For this review, take the finished solid that the model builds, in its own axes (mm). A direction names the side the tool comes from. Give positions to 0.01 mm unless a question says otherwise; leave off trailing zeros. Loops run counter-clockwise (first coordinate to the right, second up) from the corner with the lowest first, then second, coordinate; pieces in that order, holes last. Notation, with made-up numbers: (30.25, 19) - (50.25, 19) arc R20 cw to (50.25, 56) - close; hole circle Ø8 at (3.5, -23.75). An arc over 180 degrees is marked (long way). Answer in a Markdown table with one row per item.
```python
from build123d import *

# Parameters (mm, degrees)
BOSS_EXTRUDE2_DEPTH = 3
EXTRUDE_1_DEPTH     = 5
EXTRUDE_2_DEPTH     = 3


with BuildPart() as part:
    # Sketch3 → Boss-Extrude2 (new body)
    with BuildSketch(Plane.XY):
        with BuildLine():
            Line((-151, 81), (151, 81))
            ThreePointArc((151, 81), (158.071067812, 78.071067812), (161, 71))
            Line((161, 71), (161, -71))
            ThreePointArc((161, -71), (158.071067812, -78.071067812), (151, -81))
            Line((151, -81), (-151, -81))
            ThreePointArc((-151, -81), (-158.071067812, -78.071067812), (-161, -71))
            Line((-161, -71), (-161, 71))
            ThreePointArc((-161, 71), (-158.071067812, 78.071067812), (-151, 81))
        make_face()
    extrude(amount=-BOSS_EXTRUDE2_DEPTH)

    # Эскиз1 → Бобышка-Вытянуть1 (add)
    with BuildSketch(Plane(origin=(0, 0, -3), x_dir=(-1, 0, 0), z_dir=(0, 0, -1))):
        with BuildLine():
            Line((-151, -79), (151, -79))
            ThreePointArc((151, -79), (156.656854249, -76.656854249), (159, -71))
            Line((159, -71), (159, 71))
            ThreePointArc((159, 71), (156.656854249, 76.656854249), (151, 79))
            Line((151, 79), (-151, 79))
            ThreePointArc((-151, 79), (-156.656854249, 76.656854249), (-159, 71))
            Line((-159, 71), (-159, -71))
            ThreePointArc((-159, -71), (-156.656854249, -76.656854249), (-151, -79))
        make_face()
    extrude(amount=EXTRUDE_1_DEPTH)

    # Эскиз2 → Бобышка-Вытянуть2 (add)
    with BuildSketch(Plane.XY):
        with BuildLine():
            Line((-164.5, 71), (-151, 71))
            Line((-151, 71), (-151, 84.5))
            ThreePointArc((-151, 84.5), (-160.545941546, 80.545941546), (-164.5, 71))
        make_face()
        with BuildLine():
            Line((164.5, -71), (151, -71))
            Line((151, -71), (151, -84.5))
            ThreePointArc((151, -84.5), (160.545941546, -80.545941546), (164.5, -71))
        make_face()
        with BuildLine():
            Line((-151, -84.5), (-151, -71))
            Line((-151, -71), (-164.5, -71))
            ThreePointArc((-164.5, -71), (-160.545941546, -80.545941546), (-151, -84.5))
        make_face()
        with BuildLine():
            Line((151, 84.5), (151, 71))
            Line((151, 71), (164.5, 71))
            ThreePointArc((164.5, 71), (160.545941546, 80.545941546), (151, 84.5))
        make_face()
    extrude(amount=-EXTRUDE_2_DEPTH)


solid = part.part
```
1. Wall thickness on line 1 (Y direction, x = -145, z = -1.25); line 2 (X direction, y = -6, z = -6.75); line 3 (Y direction, x = -74, z = -4.5): over which ranges is each line inside the solid? List them lowest first. Write a range as [from, to].
Values:
| item | result |
|---|---|
| line 1 | y = [-81, 81] |
| line 2 | x = [-159, 159] |
| line 3 | y = [-79, 79] |
2. We need section A-A, the plane z = -1.75. Give the boundary of the cut face in (x, y), and give its area (3 significant figures).
Values:
| item | result |
|---|---|
| outline | (-164.5, -71) arc R13.5 ccw to (-151, -84.5) - (-151, -81) - (151, -81) - (151, -84.5) arc R13.5 ccw to (164.5, -71) - (161, -71) - (161, 71) - (164.5, 71) arc R13.5 ccw to (151, 84.5) - (151, 81) - (-151, 81) - (-151, 84.5) arc R13.5 ccw to (-164.5, 71) - (-161, 71) - (-161, -71) - close |
| area | 52,300 mm^2 |
3. Clearance check with flat-ended pins moving along their axes: pin 1 (1.5 mm diameter, centred on y = -82, z = -1, fed in from +X); pin 2 (2.5 mm diameter, centred on x = -162, z = -1, fed in from -Y); pin 3 (1.5 mm diameter, centred on y = 82.5, z = -2, fed in from -X). State where each tip first meets the part, or that it passes through.
Values:
| item | result |
|---|---|
| pin 1 | stops at x = 159.79 |
| pin 2 | stops at y = -80.34 |
| pin 3 | stops at x = -159.17 |
4. We need section B-B, the plane y = 22.5. Give the boundary of the cut face in (x, z), and give its area (3 significant figures).
Values:
| item | result |
|---|---|
| outline | (-161, -3) - (-159, -3) - (-159, -8) - (159, -8) - (159, -3) - (161, -3) - (161, 0) - (-161, 0) - close |
| area | 2,560 mm^2 |
5. For faces 1 (the face through (-156.594, -76.719, -5.465)), 2 (the face through (156.719, -76.594, -5.465)), 3 (the face through (-156.719, 76.594, -5.465)), list the 3-axis set-ups (+Z, -Z, +X, -X, +Y, -Y) from which the entire face can be reached by the end or side of a thin tool; tool diameter is ignored.
Values:
| item | result |
|---|---|
| face 1 | -Z, -X, -Y |
| face 2 | -Z, +X, -Y |
| face 3 | -Z, -X, +Y |
6. We need section C-C, the plane x = -11.5. Give the boundary of the cut face in (y, z).
Values:
| item | result |
|---|---|
| outline | (-81, -3) - (-79, -3) - (-79, -8) - (79, -8) - (79, -3) - (81, -3) - (81, 0) - (-81, 0) - close |
